from build123d import *

# Parameters (mm, degrees)
BOSS_EXTRUDE1_START = -11.35
SKETCH2_R           = 2
BOSS_EXTRUDE1_DEPTH = 4.15
CUT_EXTRUDE1_START  = -15.5
SKETCH2_3_R         = 3
SKETCH2_3_R_2       = 2
CUT_EXTRUDE1_DEPTH  = 2.65
CUT_EXTRUDE2_START  = -12.85
SKETCH2_4_R         = 2
CUT_EXTRUDE2_DEPTH  = 1.5
CUT_EXTRUDE3_START  = -14.85
SKETCH2_5_R         = 3
CUT_EXTRUDE3_DEPTH  = 3.5


with BuildPart() as part:
    # Sketch2 → Boss-Extrude1 (new body)
    with BuildSketch(Plane(origin=(0, 0, 0), x_dir=(0, 0, -1), z_dir=(1, 0, 0)).offset(BOSS_EXTRUDE1_START)):
        with BuildLine():
            Line((24.941275851, 120.517105669), (3.941275851, -0.682894331))
            ThreePointArc((3.941275851, -0.682894331), (-0.682894331, -3.941275851), (-3.941275851, 0.682894331))
            Line((-3.941275851, 0.682894331), (17.058724149, 121.882894331))
            ThreePointArc((17.058724149, 121.882894331), (21.682894331, 125.141275851), (24.941275851, 120.517105669))
        make_face()
        Circle(SKETCH2_R, mode=Mode.SUBTRACT)
    extrude(amount=-BOSS_EXTRUDE1_DEPTH)

    # Sketch2<3> → Cut-Extrude1 (cut)
    # profile 1 of 2: a face of its own
    with BuildSketch(Plane(origin=(0, 0, 0), x_dir=(0, 0, -1), z_dir=(1, 0, 0)).offset(CUT_EXTRUDE1_START)):
        with Locations((21, 121.2)):
            Circle(SKETCH2_3_R)
        with Locations((21, 121.2)):
            Circle(SKETCH2_3_R_2, mode=Mode.SUBTRACT)
    # profile 2 of 2: a face of its own
    with BuildSketch(Plane(origin=(0, 0, 0), x_dir=(0, 0, -1), z_dir=(1, 0, 0)).offset(CUT_EXTRUDE1_START)):
        with Locations((21, 121.2)):
            Circle(SKETCH2_3_R_2)
    extrude(amount=CUT_EXTRUDE1_DEPTH, mode=Mode.SUBTRACT)

    # Sketch2<4> → Cut-Extrude2 (cut)
    with BuildSketch(Plane(origin=(0, 0, 0), x_dir=(0, 0, -1), z_dir=(1, 0, 0)).offset(CUT_EXTRUDE2_START)):
        with Locations((21, 121.2)):
            Circle(SKETCH2_4_R)
    extrude(amount=CUT_EXTRUDE2_DEPTH, mode=Mode.SUBTRACT)

    # Sketch2<5> → Cut-Extrude3 (cut)
    with BuildSketch(Plane(origin=(0, 0, 0), x_dir=(0, 0, -1), z_dir=(1, 0, 0)).offset(CUT_EXTRUDE3_START)):
        Circle(SKETCH2_5_R)
    extrude(amount=CUT_EXTRUDE3_DEPTH, mode=Mode.SUBTRACT)


solid = part.part
CAD build for the part. Positions are in the model's coordinates, mm. A direction names the side the tool comes from. Coordinates: 2 decimals unless noted, no trailing zeros. Loops run counter-clockwise (first coordinate to the right, second up) from the corner with the lowest first, then second, coordinate; pieces in that order, holes last. Notation, with made-up numbers: (84.25, 89) - (93.25, 89) arc R13 ccw to (93.25, 107) - close; hole circle Ø10 at (83, -29). An arc over 180 degrees is marked (long way). Write item = value, one per line. Start each with the question number.
Q1. Cut at A-A, the plane z = 0. List the corners of the cut face in (x, y).
Q2. Drill centre lines: L1, parallel to Z at x = -12.35, y = 58; L2, parallel to Z at x = -12, y = 24.5. Where is each one in solid material? Low to high.
Q3. Cut at D-D, the plane y = 81. List the corners of the cut face in (x, z), then the cut area to 3 significant figures.
Q4. Pull direction Z, two halves, no side cores. Call faces 1 (the flat face through (-13.4, 60.77, -14.59)), 2 (the cylindrical face through (-12.11, 123.183, -20.74)), 3 (the flat face through (-15.5, 61, -7)): pulls with the +Z half, pulls with the -Z half, needs draft (parallel to the pull), parting line crosses it, or undercut.
Q5. Flat gauge pins, fed straight in: pin 1 Ø1.8 at (y, z) = (122.5, -22) entering from -X; pin 2 Ø2 at (x, y) = (-14.5, 104) entering from -Z; pin 3 Ø5.5 at (y, z) = (0, 0) entering from +X. Where does each tip first touch, or does it go through?
Q6. Which spindle directions (+Z, -Z, +X, -X, +Y, -Y) get a long thin tool onto all of the face, cutting with end or side? Do faces 4 (the cylindrical face through (-13, 0, 3)), 5 (the flat face through (-13.4, 60.43, -6.41)), 6 (the flat face through (-12.85, 119, -22)). Say none if no direction does.
Q7. Cut at C-C, the plane z = -21. List the corners of the cut face in (x, y).
Q8. Cut at B-B, the plane x = -13.6. List the corners of the cut face in (y, z), then the cut area to 3 significant figures.
Computed:
q1.outline = (-15.5, -4) - (-11.35, -4) - (-11.35, -3) - (-14.85, -3) - (-14.85, -2) - (-15.5, -2) - close; (-15.5, 2) - (-14.85, 2) - (-14.85, 3) - (-11.35, 3) - (-11.35, 23.43) - (-15.5, 23.43) - close
q2.L1 = -14.11 to -5.99
q2.L2 = -8.3 to -0.19
q3.outline = (-15.5, -18.09) - (-11.35, -18.09) - (-11.35, -9.98) - (-15.5, -9.98) - close
q3.area = 33.7 mm²
q4.face_1 = pulls with the -Z half
q4.face_2 = undercut
q4.face_3 = needs draft
q5.pin_1 = -12.85
q5.pin_2 = -22.25
q5.pin_3 = -14.85
q6.face_4 = +X
q6.face_5 = +Z, +X, -X, +Y
q6.face_6 = -X
q7.outline = (-15.5, 97.77) - (-11.35, 97.77) - (-11.35, 119.2) - (-12.85, 119.2) - (-12.85, 118.2) - (-15.5, 118.2) - close; (-15.5, 124.2) - (-12.85, 124.2) - (-12.85, 123.2) - (-11.35, 123.2) - (-11.35, 125.2) - (-15.5, 125.2) - close
q8.outline = (-0.68, -3.94) - (120.52, -24.94) arc R4 ccw to (121.88, -17.06) - (0.68, 3.94) arc R4 ccw to start; hole circle Ø6 at (0, 0); hole circle Ø6 at (121.2, -21)
q8.area = 978 mm²
